Build history of the part. All positions in model axes, mm. A direction names the side the tool comes from. Round coordinates to 2 decimals unless told otherwise and drop trailing zeros. Loops run counter-clockwise (first coordinate to the right, second up) from the corner with the lowest first, then second, coordinate; pieces in that order, holes last. Notation, with made-up numbers: (88, 59) -> (145, 59) arc R15 cw to (145, 69) -> close; hole circle Ø3 at (-19, -38). An arc over 180 degrees is marked (long way). Put each result on its own line as item: value. Start each with the question number.
Item 1: Cut at C-C, the plane x = 29. List the corners of the cut face in (y, z) (3 decimals).
Item 2: Cut at B-B, the plane z = -22. List the corners of the cut face in (x, y) (3 decimals).
Item 3: Cut at A-A, the plane y = 31. List the corners of the cut face in (x, z).
Item 4: Drill centre lines: probe 1 along Z at (x, y) = (11, 28); probe 2 along X at (y, z) = (17, 17.5); probe 3 along X at (y, z) = (30.75, 7.5). Where is each one in solid material? Low to high. Write a range as [from, to].
Item 5: Cut at D-D, the plane y = 17. List the corners of the cut face in (x, z).
Item 6: Pull direction X, two halves, no side cores. Call faces 5 (the flat face through (19, 29.375, 5)), 6 (the flat face through (38, 20, -10)), 7 (the flat face through (19, 10.375, -10)), 8 (the flat face through (19, 14, 12.5)): +X half, -X half, draft (parallel to the pull), parting line (faces both ways), or undercut.
Item 7: Flat gauge pins, fed straight in: pin 1 Ø4 at (x, z) = (22.5, -24.5) entering from +Y (3 decimals); pin 2 Ø2.5 at (x, y) = (19, 16.5) entering from +Z; pin 3 Ø1 at (x, y) = (11, 27) entering from +Z; pin 4 Ø6 at (x, z) = (19, 16) entering from -Y. Where does each tip first touch, or does it go through?
Item 8: Tool access for faces 1 (the flat face through (19, 24.375, -9)), 2 (the flat face through (8, 32, 5)), 3 (the flat face through (12, 14, 18)), 4 (the flat face through (19, 24, 8.5)): list every direction of +Z, -Z, +X, -X, +Y, -Y with a clear straight run to the whole face (end or side of a thin tool).
```python
from build123d import *

# Parameters (mm, degrees)
BOSS_EXTRUDE1_DEPTH = 38
SKETCH2_W           = 22
SKETCH2_H           = 10
CUT_EXTRUDE1_DEPTH  = 72.593579496
SKETCH3_W           = 14
SKETCH3_H           = 20
CUT_EXTRUDE2_DEPTH  = 59.5


with BuildPart() as part:
    # Sketch1 → Boss-Extrude1 (new body)
    with BuildSketch(Plane(origin=(0, 0, 0), x_dir=(0, 0, -1), z_dir=(1, 0, 0))):
        Polygon((41.5, 10.375), (-22.5, 10.375), (-22.5, 18.375), (-8.5, 18.375), (-8.5, 34.375), (-0.5, 34.375), (-0.5, 24.375), (19.5, 24.375), (19.5, 34.375), (27.5, 34.375), (27.5, 18.375), (41.5, 18.375), align=None)
    extrude(amount=BOSS_EXTRUDE1_DEPTH)

    # Sketch2 → Cut-Extrude1 (cut, through all)
    with BuildSketch(Plane.XY.offset(8.5)):
        with Locations((19, 34.375)):
            Rectangle(SKETCH2_W, SKETCH2_H)
    extrude(amount=-CUT_EXTRUDE1_DEPTH, mode=Mode.SUBTRACT)

    # Sketch3 → Cut-Extrude2 (cut, through all)
    with BuildSketch(Plane(origin=(0, 18.375, 0), x_dir=(1, 0, 0), z_dir=(0, 1, 0))):
        with Locations((19, -22.5)):
            Rectangle(SKETCH3_W, SKETCH3_H)
    extrude(amount=-CUT_EXTRUDE2_DEPTH, mode=Mode.SUBTRACT)


solid = part.part
```
Reply:
1. outline: (10.375, -41.5) -> (18.375, -41.5) -> (18.375, -27.5) -> (29.375, -27.5) -> (29.375, -19.5) -> (24.375, -19.5) -> (24.375, 0.5) -> (29.375, 0.5) -> (29.375, 8.5) -> (18.375, 8.5) -> (18.375, 22.5) -> (10.375, 22.5) -> close
2. outline: (0, 10.375) -> (38, 10.375) -> (38, 34.375) -> (30, 34.375) -> (30, 29.375) -> (8, 29.375) -> (8, 34.375) -> (0, 34.375) -> close
3. outline: (0, -27.5) -> (8, -27.5) -> (8, -19.5) -> (0, -19.5) -> close; (0, 0.5) -> (8, 0.5) -> (8, 8.5) -> (0, 8.5) -> close; (30, -27.5) -> (38, -27.5) -> (38, -19.5) -> (30, -19.5) -> close; (30, 0.5) -> (38, 0.5) -> (38, 8.5) -> (30, 8.5) -> close
4. probe 1: z = [-27.5, -19.5], [0.5, 8.5]
4. probe 2: x = [0, 12], [26, 38]
4. probe 3: x = [0, 8], [30, 38]
5. outline: (0, -41.5) -> (38, -41.5) -> (38, 22.5) -> (26, 22.5) -> (26, 12.5) -> (12, 12.5) -> (12, 22.5) -> (0, 22.5) -> close
6. face 5: undercut
6. face 6: +X half
6. face 7: draft
6. face 8: undercut
7. pin 1: stops at y = 29.375
7. pin 2: stops at z = 12.5
7. pin 3: stops at z = 8.5
7. pin 4: passes through
8. face 1: +X, -X, +Y
8. face 2: +Z, -Z, +Y
8. face 3: +Z, +Y, -Y
8. face 4: +Z, +X, -X, +Y
